Autodesk Inventor part; units mm, degrees
ref_plane "YZ Plane" through (0, 0, 0) normal (1, 0, 0) x (0, 1, 0)
ref_plane "XZ Plane" through (0, 0, 0) normal (0, 1, 0) x (-1, 0, 0)
ref_plane "XY Plane" through (0, 0, 0) normal (0, 0, 1) x (1, 0, 0)
sketch "Sketch1" plane through (0, 0, 0) normal (0, 0, 1) x (1, 0, 0)
  circle A0 centre (0, 0) radius 15
  circle A1 centre (0, 0) radius 55
  line L0 (15, 0) -> (55, 0) construction
  circle A2 centre (35, 0) radius 20 construction
  circle A3 centre (-17.5, 30.3109) radius 20 construction
  circle A4 centre (-17.5, -30.3109) radius 20 construction
  line L1 (0, 0) -> (-10.834, 10.3742)
  line L2 (0, 0) -> (27.5, -47.6314)
  line L3 (0, 0) -> (-55, 0) construction
  line L4 (0, 0) -> (27.5, 47.6314)
  line L5 (17.5, 30.3109) -> (27.5, 47.6314) construction
  line L6 (-1.4324, 18.1475) -> (18.5676, 52.7885) construction
  line L7 (18.5676, 52.7885) -> (36.4324, 42.4743) construction
  line L8 (36.4324, 42.4743) -> (16.4324, 7.8333) construction
  line L9 (16.4324, 7.8333) -> (-1.4324, 18.1475) construction
  line L10 (-1.4324, 18.1475) -> (36.4324, 42.4743) construction
  line L11 (18.5676, 52.7885) -> (16.4324, 7.8333) construction
  line L12 (-1.4891, -18.1802) -> (18.5109, -52.8212) construction
  line L13 (18.5109, -52.8212) -> (36.4891, -42.4416) construction
  line L14 (36.4891, -42.4416) -> (16.4891, -7.8006) construction
  line L15 (16.4891, -7.8006) -> (-1.4891, -18.1802) construction
  line L16 (-1.4891, -18.1802) -> (36.4891, -42.4416) construction
  line L17 (18.5109, -52.8212) -> (16.4891, -7.8006) construction
  line L18 (-55.0081, 10.3109) -> (-15, 10.3109) construction
  line L19 (-15, 10.3109) -> (-15, -10.3109) construction
  line L20 (-15, -10.3109) -> (-55.0081, -10.3109) construction
  line L21 (-55.0081, -10.3109) -> (-55.0081, 10.3109)
  line L22 (-55.0081, 10.3109) -> (-15, -10.3109) construction
  line L23 (-15, 10.3109) -> (-55.0081, -10.3109) construction
  line L24 (-39.1178, -2.5) -> (-30.8902, -2.5) construction
  line L25 (-30.8902, -2.5) -> (-30.8902, 2.5) construction
  line L26 (-30.8902, 2.5) -> (-39.1178, 2.5) construction
  line L27 (-39.1178, 2.5) -> (-39.1178, -2.5) construction
  line L28 (-39.1178, -2.5) -> (-30.8902, 2.5) construction
  line L29 (-30.8902, -2.5) -> (-39.1178, 2.5) construction
  line L30 (-55.0081, 10.3109) -> (-55.0081, -10.3109) construction
  line L31 (-55.0081, 10.3109) -> (-55.0081, -10.3109) construction
  circle A5 centre (0, 0) radius 5
  arc A6 (-46.1231, 28.4056) -> (-10.834, 10.3742) centre (-24.6951, 26.7945) ccw
  line L32 (-15, -10.3109) -> (-10.8943, -10.3109)
  line L33 (-46.6952, 28.5525) -> (-52.5923, 15.6119)
  arc A7 (-46.1231, 28.4056) -> (-46.6952, 28.5525) centre (-46.4222, 28.4281) ccw
  arc A8 (-52.5567, 13.8792) -> (-17.5, -10.3109) centre (-12.7886, 34.0144) ccw
  arc A9 (-17.5, -10.3109) -> (-15, -10.3109) centre (-16.25, 36.3845) ccw
  arc A10 (-52.5923, 15.6119) -> (-52.5567, 13.8792) centre (-50.7724, 14.7826) ccw
  arc A11 (-1.5384, -54.1465) -> (-3.5673, -14.5696) centre (-10.8572, -34.7838) ccw
  circle A12 centre (0, 0) radius 55
  line L34 (-1.3796, -54.7155) -> (12.7758, -53.3523)
  arc A13 (14.2587, -52.455) -> (17.6795, -10) centre (-23.063, -28.0825) ccw
  arc A14 (12.7758, -53.3523) -> (14.2587, -52.455) centre (12.5841, -51.3615) ccw
  arc A15 (-1.5384, -54.1465) -> (-1.3796, -54.7155) centre (-1.4083, -54.4169) ccw
  line L35 (16.4295, -7.8349) -> (14.3766, -4.2793)
  arc A16 (17.6795, -10) -> (16.4295, -7.8349) centre (-23.3849, -32.2652) ccw
  circle A17 centre (0, 0) radius 15
  arc A18 (47.6615, 25.741) -> (14.4013, 4.1954) centre (35.5523, 7.9893) ccw
  circle A19 centre (0, 0) radius 55
  line L36 (48.0748, 26.163) -> (39.8165, 37.7403)
  arc A20 (38.2981, 38.5759) -> (-0.1795, 20.3109) centre (35.8517, -5.9319) ccw
  arc A21 (39.8165, 37.7403) -> (38.2981, 38.5759) centre (38.1883, 36.5789) ccw
  arc A22 (47.6615, 25.741) -> (48.0748, 26.163) centre (47.8305, 25.9888) ccw
  line L37 (-1.4295, 18.1458) -> (-3.4823, 14.5902)
  arc A23 (-0.1795, 20.3109) -> (-1.4295, 18.1458) centre (39.6349, -4.1193) ccw
  circle A24 centre (0, 0) radius 15
  point P0 (-27.5, 47.6314)
  point P1 (-27.5, -47.6314)
  point P2 (17.5, -30.3109)
  point P3 (-35.004, 0)
  point P4 (-45.8939, 30.3109)
  point P5 (-52.9855, 14.7493)
  point P6 (-52.9855, 14.7493)
  point P7 (-27.5, 47.6314)
  point P8 (27.5, 47.6314)
  point P9 (27.5, -47.6314)
  point P10 (-55, 0)
  point P11 (-3.3031, -54.9007)
  point P12 (13.7195, -53.2614)
  point P13 (-7.5, 12.9904)
  point P14 (-27.5, -47.6314)
  point P15 (-55, 0)
  point P16 (27.5, 47.6314)
  point P17 (27.5, -47.6314)
  point P18 (49.1969, 24.5898)
  point P19 (39.266, 38.5121)
  point P20 (-7.5, -12.9904)
  point P21 (7.5, -12.9904)
  point P22 (-3.5673, -14.5696)
  point P23 (14.4013, 4.1954)
  dimension "d0" = 30
  dimension "d1" = 40
  dimension "d4" = 360
  dimension "d6" = 5
  dimension "d11" = 10
  dimension "d14" = 0.3
  dimension "d24" = 2
  dimension "d27" = 360
extrude "Extrusion1" add sketch "Sketch1" along normal blind 10 contours A0 L2 A5 L4 | A0 L4 A20 A21 L36 A22 A18 | L35 A16 A13 L2 A0 | L4 A5 L1 A0 | A0 L37 A23 A20 L4 | L2 A13 A14 L34 A15 A11 A0 | A0 L1 A5 L2 | A0 L32 A9 A8 A10 L33 A7 A6
properties part number "Combine mk3"
Model file for the job. Use its own axes, mm. A direction names the side the tool comes from. Give positions to 0.01 mm unless a question says otherwise; leave off trailing zeros. Order: outer loops, then holes, each group sorted by start corner. A loop starts at its lowest first (then second) coordinate and runs counter-clockwise, first axis right, second up. Notation, with made-up numbers: (17.25, 75) -> (70.25, 75) arc R27 cw to (70.25, 114) -> close; hole circle Ø6 at (11, 36). An arc over 180 degrees is marked (long way). Use CSV: the item, a comma, the result in double quotes.
1. Drop flat-ended pins along their axis: pin 1 (4.5 mm diameter, centred on x = -12.5, z = 7, fed in from -Y); pin 2 (6 mm diameter, centred on y = 6.5, z = 4, fed in from -X); pin 3 (5 mm diameter, centred on x = -42, z = 3.5, fed in from +Y). Give the stop position or say it passes through.
Outcome:
pin 1,"y = -10.95"
pin 2,"x = -50.02"
pin 3,"y = 18.46"
2. Band-saw the part on B-B, the plane y = 0. Give the cut face in (x, z).
Outcome:
outline,"(-41.6, 0) -> (-5, 0) -> (-5, 10) -> (-41.6, 10) -> close; (5, 0) -> (15, 0) -> (15, 10) -> (5, 10) -> close"
3. Band-saw the part on C-C, the plane x = 30.5. Give the cut face in (y, z), then the cut area to 3 significant figures.
Outcome:
outline,"(28.88, 0) -> (38.32, 0) -> (38.32, 10) -> (28.88, 10) -> close"
area,"94.5 mm²"
4. 3-axis set-ups, long thin cutter, end or side, ignore diameter. For faces 1 (the flat face through (15.417, -6.082, 4.93)), 2 (the flat face through (5.599, -54.043, 4.93)), 3 (the flat face through (-2.442, 16.393, 4.93)), 4 (the flat face through (-49.602, 22.173, 4.93)): which of +Z, -Z, +X, -X, +Y, -Y reach the whole face in a straight line?
Outcome:
face 1,"+Z, -Z, +X"
face 2,"+Z, -Z, +X, -Y"
face 3,"+Z, -Z, +Y"
face 4,"+Z, -Z, -X, +Y"
5. Band-saw the part on D-D, the plane y = -44.5. Give the cut face in (x, z).
Outcome:
outline,"(8.31, 0) -> (18.38, 0) -> (18.38, 10) -> (8.31, 10) -> close"
6. Mould opens along Y. For faces 5 (the cylindrical face through (17.06, -8.89, 4.93)), 6 (the flat face through (-3, 6, 0)), 7 (the cylindrical face through (-16.232, -10.328, 4.93)) say: +Y half, -Y half, draft (parallel to the pull), parting line (faces both ways), or undercut.
Outcome:
face 5,"undercut"
face 6,"draft"
face 7,"-Y half"
7. Drill centre lines: line 1 along Y through (x, z) = (0, 3); line 2 along X through (y, z) = (27.5, 3.5); line 3 along X through (y, z) = (0, 5.25). Where is each one in solid material? Low to high. Write a range as from..to.
Outcome:
line 1,"-54.58..-53.33, -16.24..-5, 5..20.56"
line 2,"-47.17..-46.17, 6.37..26.55, 44.56..47.12"
line 3,"-41.6..-5, 5..15"
